from build123d import *

# Parameters (mm, degrees)
PAD015_DEPTH   = 19
PAD016_DEPTH   = 16
THICKNESS001_T = -2.5


with BuildPart() as part:
    # Sketch039 → Pad015 (new body)
    with BuildSketch(Plane.YZ):
        with BuildLine():
            Line((56.9812455945, -19.1666932293), (85.3849313131, 115.5624248602))
            ThreePointArc((85.3849313131, 115.5624248602), (83.5681124, 123.0886932914), (76.5785062018, 126.4190014838))
            Line((76.5785062018, 126.4190014838), (36.5746674209, 126.4190014838))
            Line((23.4661256961, 64.2403714455), (36.5746674209, 126.4190014838))
            Line((7.1160182593, 67.687312386), (23.4661256961, 64.2403714455))
            Line((2.577719846, 46.1604954473), (7.1160182593, 67.687312386))
            Line((18.9278272829, 42.7135545068), (2.577719846, 46.1604954473))
            Line((8.0566616429, -8.8523786537), (18.9278272829, 42.7135545068))
            Line((56.9812455945, -19.1666932293), (8.0566616429, -8.8523786537))
        make_face()
    extrude(amount=PAD015_DEPTH)

    # Sketch040 (on Face11 of Pad015) → Pad016 (join)
    with BuildSketch(Plane.YZ.offset(19)):
        with BuildLine():
            Line((73.0077538223, 56.8529241183), (85.3849313131, 115.5624248602))
            ThreePointArc((85.3849313131, 115.5624248602), (83.5681124, 123.0886932914), (76.5785062018, 126.4190014838))
            Line((76.5785062018, 126.4190014838), (36.5746674209, 126.4190014838))
            Line((36.5746674209, 126.4190014838), (24.0831698707, 67.1672386939))
            Line((24.0831698707, 67.1672386939), (73.0077538223, 56.8529241183))
        make_face()
    extrude(amount=PAD016_DEPTH)

    # Thickness001
    thickness001_openings = [part.faces().sort_by_distance(p)[0] for p in [
        (0, 45.798185, 55.874797),
        (9.5, 32.518954, -14.009536),
    ]]
    offset(amount=THICKNESS001_T, openings=thickness001_openings)


with BuildPart() as part_1:
    # Body007 placement: moved
    add(part.part.moved(Location((3, 0, 0))))


solid = part_1.part
Design review of the part built by this model. Coordinates are the model's own, in mm. A direction names the side the tool comes from. Coordinates: 2 decimals unless noted, no trailing zeros. Order: outer loops, then holes, each group sorted by start corner. A loop starts at its lowest first (then second) coordinate and runs counter-clockwise, first axis right, second up. Notation, with made-up numbers: M -28,64 L 11,64 A5 ccw 11,68 Z; hole C -17,-31 d5. An arc over 180 degrees is marked long. Use a Markdown table: item, result.
(1) Add section A-A (x = 28). Give the boundary of the cut face in (y, z).
Worked answers:
| item | result |
|---|---|
| outline | M 24.08,67.17 L 73.01,56.85 L 85.38,115.56 A9 ccw 76.58,126.42 L 36.57,126.42 Z; hole M 27.05,69.1 L 71.08,59.81 L 82.94,116.08 A6.5 ccw 76.58,123.92 L 38.6,123.92 Z |
(2) For faces 1 (the flat face through (3, 29, 81)), 2 (the flat face through (12.367, 10.867, 44.413)), 3 (the flat face through (11.13, 15.86, 16.05)), 4 (the cylindrical face through (20.213, 49.214, 63.656)), 5 (the flat face through (12.367, 4.815, 56.773)), list the 3-axis set-ups (+Z, -Z, +X, -X, +Y, -Y) from which the entire face can be reached by the end or side of a thin tool; tool diameter is ignored.
Worked answers:
| item | result |
|---|---|
| face 1 | +Z, -Z, -X, +Y, -Y |
| face 2 | +X, -X, -Y |
| face 3 | -Z, -X |
| face 4 | -X |
| face 5 | +Z, +X, -X, -Y |
(3) Wall thickness on probe 1 along X at (y, z) = (30, 24); probe 2 along Y at (x, z) = (33, 74.5); probe 3 along Y at (x, z) = (35, 117.5): over which ranges is each line inside the solid? List them lowest first.
Worked answers:
| item | result |
|---|---|
| probe 1 | x = 19.5 to 22 |
| probe 2 | y = 25.63 to 28.18, 74.17 to 76.73 |
| probe 3 | y = 34.69 to 37.25, 83.08 to 85.58 |
(4) Add section D-D (z = 32). Give the boundary of the cut face in (x, y), then the cut area to 3 significant figures.
Worked answers:
| item | result |
|---|---|
| outline | M 3,16.67 L 22,16.67 L 22,67.77 L 3,67.77 L 3,65.21 L 19.5,65.21 L 19.5,19.22 L 3,19.22 Z |
| area | 212 mm2 |
(5) Add section B-B (x = 9). Give the boundary of the cut face in (y, z).
Worked answers:
| item | result |
|---|---|
| outline | M 2.58,46.16 L 18.93,42.71 L 8.06,-8.85 L 10.5,-9.37 L 21.37,42.2 A2.5 ccw 19.44,45.16 L 5.54,48.09 L 9.05,64.73 L 22.95,61.79 A2.5 ccw 25.91,63.72 L 38.6,123.92 L 76.58,123.92 A6.5 cw 82.94,116.08 L 54.54,-18.65 L 56.98,-19.17 L 85.38,115.56 A9 ccw 76.58,126.42 L 36.57,126.42 L 23.47,64.24 L 7.12,67.69 Z |
(6) Draft analysis for pull direction Z (two halves, no side actions). For faces 6 (the flat face through (20.26, 30.11, 95.76)), 7 (the cylindrical face through (11.37, 24.85, 62.16)), 8 (the flat face through (38, 54, 92)), 9 (the flat face through (11.134, 12.589, 46.605)), state which applies: released by +Z, released by -Z, zero draft, split by the parting line, or undercut.
Worked answers:
| item | result |
|---|---|
| face 6 | released by +Z |
| face 7 | released by -Z |
| face 8 | zero draft |
| face 9 | undercut |
(7) Add section C-C (z = 110.5). Give the boundary of the cut face in (x, y).
Worked answers:
| item | result |
|---|---|
| outline | M 3,33.22 L 38,33.22 L 38,84.32 L 3,84.32 L 3,81.76 L 35.5,81.76 L 35.5,35.77 L 3,35.77 Z |
(8) For P1, Ø6, axis at x = 30, z = 69.5, coming from the -Y side; P2, Ø17, axis at y = 61.5, z = 76.5, coming from the -X side; P3, Ø1, axis at x = 12, z = 28, coming from the +Y side; P4, Ø12, axis at y = 23, z = 47.5, coming from the -X side, all flat-tipped, find the tip position at first contact; note any pin that passes through.
Worked answers:
| item | result |
|---|---|
| P1 | stops at y = 24.08 |
| P2 | stops at x = 35.5 |
| P3 | stops at y = 67.03 |
| P4 | stops at x = 3 |
